Source: CAD feature listing. Evaluate the final solid. Frame: model axes, mm. A direction names the side the tool comes from. Round coordinates to 2 decimals unless told otherwise and drop trailing zeros. Loops run counter-clockwise (first coordinate to the right, second up) from the corner with the lowest first, then second, coordinate; pieces in that order, holes last. Notation, with made-up numbers: (-20.75, -18) -> (38.25, -18) arc R21 cw to (38.25, -4) -> close; hole circle Ø10 at (-32, 79.5). An arc over 180 degrees is marked (long way). Put each result on its own line as item: value. Start each with the question number.
1. Contact query for flat-ended pins moving along their axis: pin 1 (6.5 mm diameter, centred on y = 10.5, z = 1.5, fed in from -X); pin 2 (8 mm diameter, centred on y = -9.5, z = -5, fed in from +X); pin 3 (3.5 mm diameter, centred on x = -14.5, z = 3.5, fed in from +Y); pin 4 (2.5 mm diameter, centred on y = 11.5, z = 2, fed in from +X). Output: stop coordinate, or through.
2. Material intervals for L1, parallel to X at y = 10, z = 4.75; L2, parallel to Y at x = -8, z = -0.5; L3, parallel to Z at x = 3.5, y = 8, sorted ascending.
3. Cut plane A-A (x = -16). Return the cut outline in (y, z), then the cut area to 3 significant figures.
4. Draft query along Z for faces 1 (the flat face through (0, -10, -7)), 2 (the cylindrical face through (-5, 6, 0)), 3 (the flat face through (9, 0, 0)). Return one class per face: pulls with the +Z half, pulls with the -Z half, needs draft (parallel to the pull), parting line crosses it, or undercut.
5. Cut plane C-C (y = 8). Return the cut outline in (x, z), then the cut area to 3 significant figures.
6. Cut plane B-B (y = 0.6). Return the cut outline in (x, z), then the cut area to 3 significant figures.
7. Cut plane D-D (z = -5). Return the cut outline in (x, y), then the cut area to 3 significant figures.
8. Set-up query: faces 4 (the flat face through (-13.6, -13.4, 1.7)), 5 (the flat face through (-0.5, 10.3, 0.1)), 6 (the flat face through (12, -13.4, 0)). Return all of +Z, -Z, +X, -X, +Y, -Y with unobstructed straight access to the full face (end or side cutting, diameter ignored); none if empty.
```python
from build123d import *

# Parameters (mm, degrees)
SKETCH_3_R          = 5
EXTRUDE_3_DEPTH     = 7
SKETCH_5_R          = 2.75
CUT_EXTRUDE_1_DEPTH = 10
SKETCH_6_W          = 1
SKETCH_6_H          = 13.139857665
CUT_EXTRUDE_2_DEPTH = 14
SKETCH_7_R          = 2
CUT_EXTRUDE_3_DEPTH = 37.405494091


with BuildPart() as part:
    # 草图3 → 凸台-拉伸3 (new, symmetric)
    with BuildSketch(Plane.XY):
        Polygon((-9, -13.4), (-21, -13.4), (-21, -19.4), (21, -19.4), (21, -13.4), (9, -13.4), (9, 13.4), (-9, 13.4), align=None)
        with Locations((0, 0.6)):
            Circle(SKETCH_3_R, mode=Mode.SUBTRACT)
    extrude(amount=EXTRUDE_3_DEPTH, both=True)

    # 草图5 → 切除-拉伸1 (cut)
    with BuildSketch(Plane(origin=(0, -13.4, 0), x_dir=(1, 0, 0), z_dir=(0, 1, 0))):
        with Locations(Location((-16, 0, 0), (0, 0, 270))):
            Circle(SKETCH_5_R)
        with Locations(Location((16, 0, 0), (0, 0, 180))):
            Circle(SKETCH_5_R)
    extrude(amount=-CUT_EXTRUDE_1_DEPTH, mode=Mode.SUBTRACT)

    # 草图6 → 切除-拉伸2 (cut)
    with BuildSketch(Plane.XY.offset(7)):
        with Locations((0, 10.029998353)):
            Rectangle(SKETCH_6_W, SKETCH_6_H)
    extrude(amount=-CUT_EXTRUDE_2_DEPTH, mode=Mode.SUBTRACT)

    # 草图7 → 切除-拉伸3 (cut, through all)
    with BuildSketch(Plane(origin=(9, 0, 0), x_dir=(0, 0, -1), z_dir=(1, 0, 0))):
        with Locations(Location((0, 8, 0), (0, 0, 90))):
            Circle(SKETCH_7_R)
    extrude(amount=-CUT_EXTRUDE_3_DEPTH, mode=Mode.SUBTRACT)


solid = part.part
```
Solution:
1. pin 1: stops at x = -9
1. pin 2: stops at x = 21
1. pin 3: stops at y = -13.4
1. pin 4: stops at x = 9
2. L1: x = -9 to -0.5, 0.5 to 9
2. L2: y = -19.4 to 6.06, 9.94 to 13.4
2. L3: z = -7 to -2, 2 to 7
3. outline: (-19.4, -7) -> (-13.4, -7) -> (-13.4, -2.75) -> (-19.4, -2.75) -> close; (-19.4, 2.75) -> (-13.4, 2.75) -> (-13.4, 7) -> (-19.4, 7) -> close
3. area: 51.0 mm^2
4. face 1: pulls with the -Z half
4. face 2: undercut
4. face 3: needs draft
5. outline: (-9, -7) -> (-0.5, -7) -> (-0.5, -2) -> (-9, -2) -> close; (-9, 2) -> (-0.5, 2) -> (-0.5, 7) -> (-9, 7) -> close; (0.5, -7) -> (9, -7) -> (9, -2) -> (0.5, -2) -> close; (0.5, 2) -> (9, 2) -> (9, 7) -> (0.5, 7) -> close
5. area: 170 mm^2
6. outline: (-9, -7) -> (-5, -7) -> (-5, 7) -> (-9, 7) -> close; (5, -7) -> (9, -7) -> (9, 7) -> (5, 7) -> close
6. area: 112 mm^2
7. outline: (-21, -19.4) -> (21, -19.4) -> (21, -13.4) -> (9, -13.4) -> (9, 13.4) -> (0.5, 13.4) -> (0.5, 5.57) arc R5 cw (long way) to (-0.5, 5.57) -> (-0.5, 13.4) -> (-9, 13.4) -> (-9, -13.4) -> (-21, -13.4) -> close
7. area: 648 mm^2
8. face 4: +Z, -Z, -X, +Y
8. face 5: +Z, -Z, +Y
8. face 6: +Z, -Z, +X, +Y
